from build123d import *

# Parameters (mm, degrees)
F1_DEPTH = 6.35
F2_SIZE  = 38.1
F3_R     = 9.525
F4_DEPTH = 6.351


with BuildPart() as f1:
    # F0 (on Top) → F1 (new body)
    with BuildSketch(Plane.XY):
        Polygon((212.344, 0), (348.488, 0), (348.488, 609.6), (212.344, 609.6), (174.244, 571.5), (136.144, 609.6), (0, 609.6), (0, 0), (136.144, 0), (174.244, 38.1), align=None)
    extrude(amount=F1_DEPTH)

    # F2
    f2_edges = [f1.edges().sort_by_distance(p)[0] for p in [
        (0, 609.6, 3.175),
        (348.488, 609.6, 3.175),
        (348.488, 0, 3.175),
        (0, 0, 3.175),
    ]]
    chamfer(f2_edges, length=F2_SIZE)

    # F3 (on face) → F4 (cut, through all)
    with BuildSketch(Plane(origin=(0, 0, 0), x_dir=(1, 0, 0), z_dir=(0, 0, -1))):
        with Locations((38.1, -571.5)):
            Circle(F3_R)
        with Locations((136.144, -571.5)):
            Circle(F3_R)
        with Locations((212.344, -571.5)):
            Circle(F3_R)
        with Locations((310.388, -571.5)):
            Circle(F3_R)
        with Locations((38.1, -38.1)):
            Circle(F3_R)
        with Locations((136.144, -38.1)):
            Circle(F3_R)
        with Locations((212.344, -38.1)):
            Circle(F3_R)
        with Locations((310.388, -38.1)):
            Circle(F3_R)
    extrude(amount=-F4_DEPTH, mode=Mode.SUBTRACT)


solid = f1.part
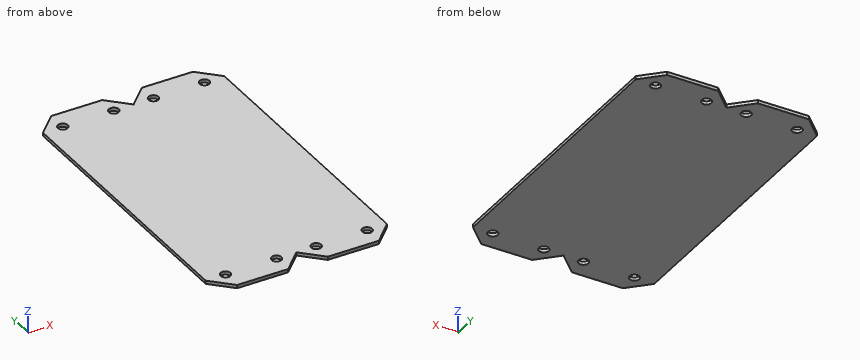
Verification items for the finished model (mm, model axes). Coordinates: 2 decimals unless noted, no trailing zeros. One line per item, written item: value.
1. Material ranges on line 1 along Y through (x, z) = (138, 5); line 2 along Y through (x, z) = (205.5, 5.75); line 3 along X through (y, z) = (564.5, 6), recorded low to high. Write a range as from..to.
Answers follow:
line 1: 1.86..28.76, 47.44..562.16, 580.84..607.74
line 2: 6.84..31.48, 44.72..564.88, 578.12..602.76
line 3: 0..31.64, 44.56..129.68, 142.6..205.88, 218.8..303.93, 316.85..348.49
2. Gauge pin test, flat ends, axial feed: P1, Ø15, axis at x = 212.344, y = 38.1, coming from the +Z side; P2, Ø22, axis at x = 38.1, y = 38.1, coming from the +Z side. Record the tip position at first contact, or that the pin passes through.
Answers follow:
P1: through
P2: z = 6.35
3. Section check A-A on z = 1. Give the number of separate pieces and of enclosed holes in the cut face, plus the area to 3 significant figures.
Answers follow:
separate pieces: 1
enclosed holes: 8
area: 204,000 mm^2
